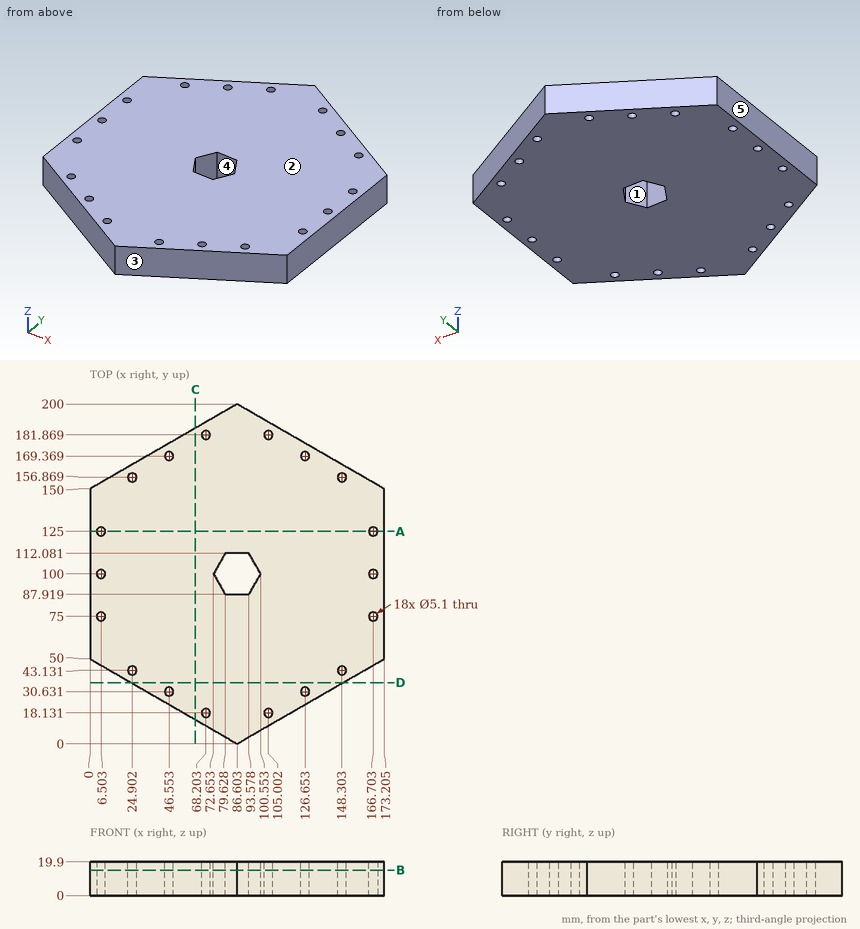
Verification items for this drawing (mm, ordinates from the low corner). A direction names the side the tool comes from. Coordinates: 2 decimals unless noted, no trailing zeros. Write each loop counter-clockwise with the first axis right and the second up, starting at its lowest first coordinate (ties: lowest second). Pieces come first, ordered by that corner, then holes. Notation, with made-up numbers: M 44.5,62 L 99.5,62 A27 cw 99.5,87 Z; hole C 5,66.5 d6. An arc over 180 degrees is marked long. One line per item, written item: value. Start each with the question number.
(1) Sectioned sample at C-C, the plane x = 62. Enter the section's corners in (y, z) (1 decimal).
(2) Sectioned sample at A-A, the plane y = 125. Enter the section's corners in (x, z) (1 decimal).
(3) Sectioned sample at D-D, the plane y = 36. Enter the section's corners in (x, z), and give its area (3 significant figures).
(4) Sectioned sample at B-B, the plane z = 15. State how many separate pieces and enclosed holes the cut face has, and give its area (3 significant figures).
(5) Tool access check on the marked faces 1 and 2. Record the directions out of +Z, -Z, +X, -X, +Y, -Y that give a thin tool (end or side, any length) a straight path to the whole face; none if there is none.
(6) Depth check by flat-ended pin: pin 1 (3 mm diameter, centred on x = 6.5, y = 125, fed in from +Z); pin 2 (3 mm diameter, centred on x = 79.5, z = 12.5, fed in from -Y) (1 decimal); pin 3 (3 mm diameter, centred on y = 32, z = 10.5, fed in from -X); pin 4 (8 mm diameter, centred on x = 103.5, z = 8.5, fed in from +Y). Enter the tip coordinate at first touch or a pass-through.
(7) Scan lines: line 1 along X through (y, z) = (125.5, 11) (1 decimal); line 2 along Y through (x, z) = (46.5, 15.25) (1 decimal); line 3 along X through (y, z) = (167.5, 14) (1 decimal). Record each from-to range of solid material in increasing order. Write a range as [from, to].
(8) Release check for a two-part mould opening along X. For the marked faces 3, 4 and 5 record: released by +X, released by -X, zero draft, split by the parting line, or undercut.
Filled sheet:
1. outline: M 14.2,0 L 185.8,0 L 185.8,19.9 L 14.2,19.9 Z
2. outline: M 0,0 L 4,0 L 4,19.9 L 0,19.9 Z; M 9.1,0 L 164.2,0 L 164.2,19.9 L 9.1,19.9 Z; M 169.3,0 L 173.2,0 L 173.2,19.9 L 169.3,19.9 Z
3. outline: M 24.25,0 L 148.96,0 L 148.96,19.9 L 24.25,19.9 Z
3. area: 2,480 mm²
4. separate pieces: 1
4. enclosed holes: 19
4. area: 25,100 mm²
5. face 1: +Z, -Z
5. face 2: +Z, +X, -X, +Y, -Y
6. pin 1: through
6. pin 2: y = 3.2
6. pin 3: x = 28.58
6. pin 4: y = 192.55
7. line 1: [0, 4], [9, 164.2], [169.2, 173.2]
7. line 2: [23.2, 28.1], [33.2, 166.8], [171.9, 176.8]
7. line 3: [30.3, 44.8], [48.3, 124.9], [128.4, 142.9]
8. face 3: released by +X
8. face 4: undercut
8. face 5: released by -X
